Read the model definition and answer for the solid it produces. Units are mm, in the model's axes. A direction names the side the tool comes from. Round coordinates to 2 decimals unless told otherwise and drop trailing zeros. Order: outer loops, then holes, each group sorted by start corner. A loop starts at its lowest first (then second) coordinate and runs counter-clockwise, first axis right, second up.
from build123d import *

# Parameters (mm, degrees)
SKETCH_1_R               = 9.17
EXTRUDE_1_DEPTH          = 11
CUT_EXTRUDE_1_REACH      = 19.005
PATTERN_CIRCULAR_1_COUNT = 20
SKETCH_3_R               = 11
EXTRUDE_2_DEPTH          = 0.5
EXTRUDE_START            = 0.5
SKETCH_4_R               = 11
EXTRUDE_3_DEPTH          = 0.5
SKETCH_5_R               = 7.5
EXTRUDE_4_DEPTH          = 10
CUT_EXTRUDE_2_REACH      = 28.944
SKETCH_6_R               = 2.5
FILLET_1_SIZE            = 0.5
FILLET_1_SIZE_2          = 3


with BuildPart() as part:
    # 草圖1 → 填料-伸長1 (new body)
    with BuildSketch(Plane.XY):
        Circle(SKETCH_1_R)
    extrude(amount=EXTRUDE_1_DEPTH)

    # 草圖2 → 除料-伸長1 (cut, up to next)
    with BuildSketch(Plane.XY.offset(11), mode=Mode.PRIVATE) as cut_extrude_1_sk1:
        with BuildLine():
            ThreePointArc((-1.117541879, 9.101648211), (0, 9.17), (1.117541879, 9.101648211))
            ThreePointArc((1.117541879, 9.101648211), (0.997261135, 8.994202524), (0.95, 8.84))
            ThreePointArc((0.95, 8.84), (0, 7.89), (-0.95, 8.84))
            ThreePointArc((-0.95, 8.84), (-0.997261135, 8.994202524), (-1.117541879, 9.101648211))
        make_face()
    cut_extrude_1_tool1 = extrude(cut_extrude_1_sk1.sketch, amount=-CUT_EXTRUDE_1_REACH, mode=Mode.PRIVATE) & part.part
    cut_extrude_1 = cut_extrude_1_tool1.solids().sort_by_distance((0, 8.608887, 11))[0]
    add(cut_extrude_1, mode=Mode.SUBTRACT)

    # 環狀複製排列1: 除料-伸長1 ×20 about axis
    pattern_circular_1_axis = Axis((0, 0, 0), (0, 0, 1))
    for i in range(1, PATTERN_CIRCULAR_1_COUNT):
        add(cut_extrude_1.rotate(pattern_circular_1_axis, i * 360 / PATTERN_CIRCULAR_1_COUNT), mode=Mode.SUBTRACT)

    # 草圖3 → 填料-伸長2 (add)
    with BuildSketch(Plane.XY.offset(11)):
        Circle(SKETCH_3_R)
    extrude(amount=EXTRUDE_2_DEPTH)

    # 草圖4 → 填料-伸長3 (add)
    with BuildSketch(Plane(origin=(0, 0, 0), x_dir=(-1, 0, 0), z_dir=(0, 0, -1)).offset(EXTRUDE_START)):
        with Locations(Location((0, 0, 0), (0, 0, 180))):
            Circle(SKETCH_4_R)
    extrude(amount=-EXTRUDE_3_DEPTH)

    # 草圖5 → 填料-伸長4 (add)
    with BuildSketch(Plane(origin=(0, 0, -0.5), x_dir=(-1, 0, 0), z_dir=(0, 0, -1))):
        Circle(SKETCH_5_R)
    extrude(amount=EXTRUDE_4_DEPTH)

    # 草圖6 → 除料-伸長2 (cut, up to next)
    with BuildSketch(Plane(origin=(0, 0, -10.5), x_dir=(-1, 0, 0), z_dir=(0, 0, -1)), mode=Mode.PRIVATE) as cut_extrude_2_sk1:
        Circle(SKETCH_6_R)
    cut_extrude_2_tool1 = extrude(cut_extrude_2_sk1.sketch, amount=-CUT_EXTRUDE_2_REACH, mode=Mode.PRIVATE) & part.part
    add(cut_extrude_2_tool1.solids().sort_by_distance((0, 0, -10.5))[0], mode=Mode.SUBTRACT)

    # 圓角1
    # an asymmetric fillet: 3, 0.5 mm, written as the material it takes off along each edge
    with BuildSketch(Plane(origin=(0, 0, -10.5), x_dir=(-1, 0, 0), z_dir=(0, -1, 0))) as fillet_1_piece_1:
        with BuildLine():
            Bezier((7.5, -FILLET_1_SIZE), (7.5, 0), (7.5 - FILLET_1_SIZE_2, 0), weights=[1, 0.707106781, 1])
            Line((7.5 - FILLET_1_SIZE_2, 0), (7.5, 0))
            Line((7.5, 0), (7.5, -FILLET_1_SIZE))
        make_face()
    revolve(axis=Axis((0, 0, -10.5), (0, 0, -1)), mode=Mode.SUBTRACT)


solid = part.part
Q1. Straight lines are drawn through the part: probe 1 along Y at (x, z) = (0, 5); probe 2 along Y at (x, z) = (0, -3.25); probe 3 along Z at (x, y) = (8.75, 4). For each, find the intervals that lie inside material, in ascending order.
Outcome:
probe 1: y = -7.89 to -2.5, 2.5 to 7.89
probe 2: y = -7.5 to -2.5, 2.5 to 7.5
probe 3: z = -0.5 to 0, 11 to 11.5
Q2. A cutting plane is placed at A-A, the plane z = -1.25. Give the vertices of the cut face in (x, y), plus the area to 3 significant figures.
Outcome:
outline: circle Ø15 at (0, 0); hole circle Ø5 at (0, 0)
area: 157 mm2
Q3. Flat-ended cylindrical pins translate along their axes: pin 1 (2 mm diameter, centred on y = -5, z = -1, fed in from -X); pin 2 (4 mm diameter, centred on x = 0, y = 0, fed in from -Z); pin 3 (2 mm diameter, centred on y = -7.5, z = 4, fed in from +X); pin 4 (4 mm diameter, centred on y = -5.5, z = -5, fed in from -X). Find the tip coordinate at first contact, or state that the pin passes through.
Outcome:
pin 1: stops at x = -10.19
pin 2: passes through
pin 3: stops at x = 6.47
pin 4: stops at x = -6.63
Q4. For a pull along Y with two mould halves and no side action, classify faces 4 (the face through (7.89, -0.02, 5.58)), 5 (the face through (0.02, 7.89, 5.58)), 6 (the face through (-0.02, -7.89, 5.58)), 7 (the face through (7.2, -2.6, -0.5)) as released by +Y, released by -Y, zero draft, split by the parting line, or undercut.
Outcome:
face 4: undercut
face 5: released by +Y
face 6: released by -Y
face 7: zero draft
Q5. For faces 1 (the face through (-7.498, 2.458, 5.577)), 2 (the face through (-2, -2, -10.5)), 3 (the face through (7.493, 0.33, -5.184)), determine the directions among +Z, -Z, +X, -X, +Y, -Y from which every point of the face is accessible in a straight line to the end or side of a thin tool.
Outcome:
face 1: none
face 2: -Z, +X, -X, +Y, -Y
face 3: -Z
